from build123d import *

# Parameters (mm, degrees)
SKETCH1_W             = 27.120418848
SKETCH1_H             = 25
BOSS_EXTRUDE2_DEPTH   = 63
SKETCH1_W_2           = 27.22513089
BOSS_EXTRUDE2_2_DEPTH = 63
BOSS_EXTRUDE3_DEPTH   = 40
SKETCH1_6_W           = 50
SKETCH1_6_H           = 27.434554974
BOSS_EXTRUDE4_DEPTH   = 40
CUT_EXTRUDE1_START    = 40
SKETCH1_7_W           = 50
SKETCH1_7_H           = 27.434554974
CUT_EXTRUDE1_DEPTH    = 19
SKETCH2_W             = 39
SKETCH2_H             = 5.946926335
CUT_EXTRUDE2_DEPTH    = 140.978569788


with BuildPart() as part:
    # Sketch1 → Boss-Extrude2 (new body)
    with BuildSketch(Plane.XY):
        with Locations((13.560209424, 12.5)):
            Rectangle(SKETCH1_W, SKETCH1_H)
    extrude(amount=BOSS_EXTRUDE2_DEPTH)



with BuildPart() as body_2:
    # Sketch1 → Boss-Extrude2 2 (new body)
    with BuildSketch(Plane.XY):
        with Locations((86.387434555, 12.5)):
            Rectangle(SKETCH1_W_2, SKETCH1_H)
    extrude(amount=BOSS_EXTRUDE2_2_DEPTH)


with BuildPart() as part_1:
    add(part.part)

    add(body_2.part)  # Boss-Extrude3 merges body 2
    # Sketch1<5> → Boss-Extrude3 (add)
    with BuildSketch(Plane.XY):
        Polygon((27.120418848, 25), (27.120418848, 0), (72.77486911, 0), (72.77486911, 25), (100, 25), (100, 75), (75, 75), (75, 47.565445026), (25, 47.565445026), (25, 75), (0, 75), (0, 25), align=None)
    extrude(amount=BOSS_EXTRUDE3_DEPTH)

    # Sketch1<6> → Boss-Extrude4 (add)
    with BuildSketch(Plane.XY):
        with Locations((50, 61.282722513)):
            Rectangle(SKETCH1_6_W, SKETCH1_6_H)
    extrude(amount=BOSS_EXTRUDE4_DEPTH)

    # Sketch1<7> → Cut-Extrude1 (cut)
    with BuildSketch(Plane.XY.offset(CUT_EXTRUDE1_START)):
        with Locations((50, 61.282722513)):
            Rectangle(SKETCH1_7_W, SKETCH1_7_H)
    extrude(amount=-CUT_EXTRUDE1_DEPTH, mode=Mode.SUBTRACT)

    # Sketch2 → Cut-Extrude2 (cut, through all)
    with BuildSketch(Plane.ZY):
        with Locations((31.5, 2.973463168)):
            Rectangle(SKETCH2_W, SKETCH2_H)
    extrude(amount=-CUT_EXTRUDE2_DEPTH, mode=Mode.SUBTRACT)


solid = part_1.part
Model file for the job. Use its own axes, mm. A direction names the side the tool comes from. Round coordinates to 2 decimals unless told otherwise and drop trailing zeros. Loops run counter-clockwise (first coordinate to the right, second up) from the corner with the lowest first, then second, coordinate; pieces in that order, holes last.
1. Band-saw the part on A-A, the plane z = 59.5. List the corners of the cut face in (x, y), and give its area (3 significant figures).
Check values:
outline: (0, 0) - (27.12, 0) - (27.12, 25) - (0, 25) - close; (72.77, 0) - (100, 0) - (100, 25) - (72.77, 25) - close
area: 1,360 mm2
2. Mould opens along Z. For faces 6 (the flat face through (49, 3, 12)), 7 (the flat face through (13, 0, 57)), 8 (the flat face through (86, 3, 51)), 9 (the flat face through (50, 61, 21)) say: +Z half, -Z half, draft (parallel to the pull), parting line (faces both ways), or undercut.
Check values:
face 6: undercut
face 7: draft
face 8: undercut
face 9: +Z half
3. Drop flat-ended pins along their axis: P1, Ø1.8, axis at x = 92, y = 3.5, coming from the -Z side; P2, Ø22, axis at x = 60, y = 60.5, coming from the +Z side; P3, Ø11.5, axis at x = 91, z = 54.5, coming from the +Y side; P4, Ø5, axis at x = 39.5, y = 3, coming from the +Z side. Give the stop position or say it passes through.
Check values:
P1: stops at z = 0
P2: stops at z = 21
P3: stops at y = 25
P4: stops at z = 12
4. Tool access for faces 1 (the flat face through (13, 3, 51)), 2 (the flat face through (13, 13, 63)), 3 (the flat face through (72.775, 12, 51)), 4 (the flat face through (86, 25, 51)), 5 (the flat face through (75, 61, 31)): list every direction of +Z, -Z, +X, -X, +Y, -Y with a clear straight run to the whole face (end or side of a thin tool).
Check values:
face 1: +X, -X, -Y
face 2: +Z, +X, -X, +Y, -Y
face 3: +Z, +Y, -Y
face 4: +Z, +X, -X, +Y
face 5: +Z, +Y
5. Band-saw the part on D-D, the plane x = 86. List the corners of the cut face in (y, z), and give its area (3 significant figures).
Check values:
outline: (0, 0) - (75, 0) - (75, 40) - (25, 40) - (25, 63) - (0, 63) - (0, 51) - (5.95, 51) - (5.95, 12) - (0, 12) - close
area: 3,340 mm2
6. Wall check: probe 1 along X at (y, z) = (9.5, 40.5); probe 2 along Z at (x, y) = (55.5, 27.5); probe 3 along X at (y, z) = (65.5, 32). Give the ranges that are in metal, low to high.
Check values:
probe 1: x = 0 to 27.12, 72.77 to 100
probe 2: z = 0 to 40
probe 3: x = 0 to 25, 75 to 100
7. Band-saw the part on B-B, the plane y = 56.5. List the corners of the cut face in (x, z), and give its area (3 significant figures).
Check values:
outline: (0, 0) - (100, 0) - (100, 40) - (75, 40) - (75, 21) - (25, 21) - (25, 40) - (0, 40) - close
area: 3,050 mm2
8. Band-saw the part on C-C, the plane z = 24.5. List the corners of the cut face in (x, y).
Check values:
outline: (0, 5.95) - (100, 5.95) - (100, 75) - (75, 75) - (75, 47.57) - (25, 47.57) - (25, 75) - (0, 75) - close
